```python
from build123d import *

# Parameters (mm, degrees)
BOSS_EXTRUDE1_DEPTH = 1.6
FILLET1_R           = 0.5
FILLET2_R           = 0.25
FILLET3_R           = 0.15
SKETCH2_R           = 1
CUT_EXTRUDE3_DEPTH  = 35.771862445
CUT_EXTRUDE4_DEPTH  = 0.5
FILLET4_R           = 0.15
FILLET5_R           = 0.05


with BuildPart() as part:
    # Sketch1 → Boss-Extrude1 (new body)
    with BuildSketch(Plane.XY):
        with BuildLine():
            Line((4.463625287, 0), (-6.536374713, 0))
            Line((-6.536374713, 0), (-6.536374713, 6))
            Line((-6.536374713, 6), (18.880501335, 6))
            ThreePointArc((18.880501335, 6), (27.540755373, 4.722813233), (35.463625287, 1))
            Line((35.463625287, 1), (5.463625287, 1))
            Line((5.463625287, 1), (4.463625287, 0))
        make_face()
    extrude(amount=BOSS_EXTRUDE1_DEPTH)

    # Fillet1
    fillet1_edges = [part.edges().sort_by_distance(p)[0] for p in [
        (35.463625287, 1, 0.8),
    ]]
    fillet(fillet1_edges, radius=FILLET1_R)

    # Fillet2
    fillet2_edges = [part.edges().sort_by_distance(p)[0] for p in [
        (4.463625287, 0, 0.8),
        (-6.536374713, 0, 0.8),
        (-6.536374713, 6, 0.8),
        (5.463625287, 1, 0.8),
    ]]
    fillet(fillet2_edges, radius=FILLET2_R)

    # Fillet3
    fillet3_edges = [part.edges().sort_by_distance(p)[0] for p in [
        (6.297063311, 6, 1.6),
        (26.691835994, 4.96520414, 0),
        (26.691835994, 4.96520414, 1.6),
        (34.195651711, 1.369811089, 0),
        (34.195651711, 1.369811089, 1.6),
        (19.640038493, 1, 0),
        (19.640038493, 1, 1.6),
        (4.963625287, 0.5, 0),
        (4.963625287, 0.5, 1.6),
        (-0.963151409, 0, 0),
        (-6.536374713, 3, 0),
        (-6.463151409, 5.926776695, 0),
        (-6.463151409, 0.073223305, 0),
        (4.455742754, 0.019030117, 0),
        (-0.963151409, 0, 1.6),
        (-6.536374713, 3, 1.6),
        (-6.463151409, 5.926776695, 1.6),
        (-6.463151409, 0.073223305, 1.6),
        (4.455742754, 0.019030117, 1.6),
        (5.471507819, 0.980969883, 0),
        (5.471507819, 0.980969883, 1.6),
        (6.297063311, 6, 0),
    ]]
    fillet(fillet3_edges, radius=FILLET3_R)

    # Sketch2 → Cut-Extrude3 (cut, through all)
    with BuildSketch(Plane.XY):
        with Locations((-2.886374713, 3.35)):
            Circle(SKETCH2_R)
    extrude(amount=CUT_EXTRUDE3_DEPTH, mode=Mode.SUBTRACT)

    # Sketch3 → Cut-Extrude4 (cut)
    with BuildSketch(Plane.XY.offset(1.6)):
        with BuildLine():
            Line((20.880501335, 5.6), (8.880501335, 5.6))
            ThreePointArc((8.880501335, 5.6), (14.880501335, 4.678784028), (20.880501335, 5.6))
        make_face()
    extrude(amount=-CUT_EXTRUDE4_DEPTH, mode=Mode.SUBTRACT)

    # Fillet4
    fillet4_edges = [part.edges().sort_by_distance(p)[0] for p in [
        (20.880501335, 5.6, 1.35),
        (8.880501335, 5.6, 1.35),
    ]]
    fillet(fillet4_edges, radius=FILLET4_R)

    # Fillet5
    fillet5_edges = [part.edges().sort_by_distance(p)[0] for p in [
        (14.880501335, 4.678784028, 1.6),
        (14.880501335, 5.6, 1.6),
        (9.804574431, 5.46876365, 1.6),
        (19.956428239, 5.46876365, 1.6),
    ]]
    fillet(fillet5_edges, radius=FILLET5_R)


solid = part.part
```
Read the model definition and answer for the solid it produces. Units are mm, in the model's axes. A direction names the side the tool comes from. Coordinates: 2 decimals unless noted, no trailing zeros. Loops run counter-clockwise (first coordinate to the right, second up) from the corner with the lowest first, then second, coordinate; pieces in that order, holes last. Notation, with made-up numbers: (-18, 70) -> (36, 70) arc R26 cw to (36, 103) -> close; hole circle Ø10 at (34.5, 9). An arc over 180 degrees is marked (long way). Return JSON: item names as keys, results as strings.
Item 1: For a pull along Y with two mould halves and no side action, classify faces 1 (the flat face through (20, 1, 1)), 2 (the flat face through (6, 6, 1)), 3 (the cylindrical face through (-3.62, 4.03, 0.79)) as +Y half, -Y half, draft (parallel to the pull), parting line (faces both ways), or undercut.
Answers:
{"face 1": "-Y half", "face 2": "+Y half", "face 3": "undercut"}
Item 2: A flat-ended cylindrical pin translates along its axis: P1, Ø1.2, axis at x = -2.89, y = 3.35, coming from the +Z side. Find the tip coordinate at first contact, or state that the pin passes through.
Answers:
{"P1": "passes through"}
Item 3: Find section A-A (z = 0.85). Determine the outline of the cut face in (x, y).
Answers:
{"outline": "(-6.54, 0.25) arc R0.25 ccw to (-6.29, 0) -> (4.36, 0) arc R0.25 ccw to (4.54, 0.07) -> (5.39, 0.93) arc R0.25 cw to (5.57, 1) -> (33.71, 1) arc R0.5 ccw to (33.96, 1.93) arc R30 ccw to (18.88, 6) -> (-6.29, 6) arc R0.25 ccw to (-6.54, 5.75) -> close; hole circle Ø2 at (-2.89, 3.35)"}
Item 4: Find the intervals of material crossed by probe 1 along Y at (x, z) = (15, 1.15); probe 2 along X at (y, z) = (3.35, 0.6); probe 3 along X at (y, z) = (3.5, 0.6), in increasing order.
Answers:
{"probe 1": "y = 1 to 4.68, 5.6 to 6", "probe 2": "x = -6.54 to -3.89, -1.89 to 31.21", "probe 3": "x = -6.54 to -3.88, -1.9 to 30.87"}
Item 5: For faces 4 (the cylindrical face through (34.2, 1.38, 0.81)), 5 (the flat face through (15, 5, 1.1)), determine the directions among +Z, -Z, +X, -X, +Y, -Y from which every point of the face is accessible in a straight line to the end or side of a thin tool.
Answers:
{"face 4": "+Z, -Z, +X", "face 5": "+Z"}
